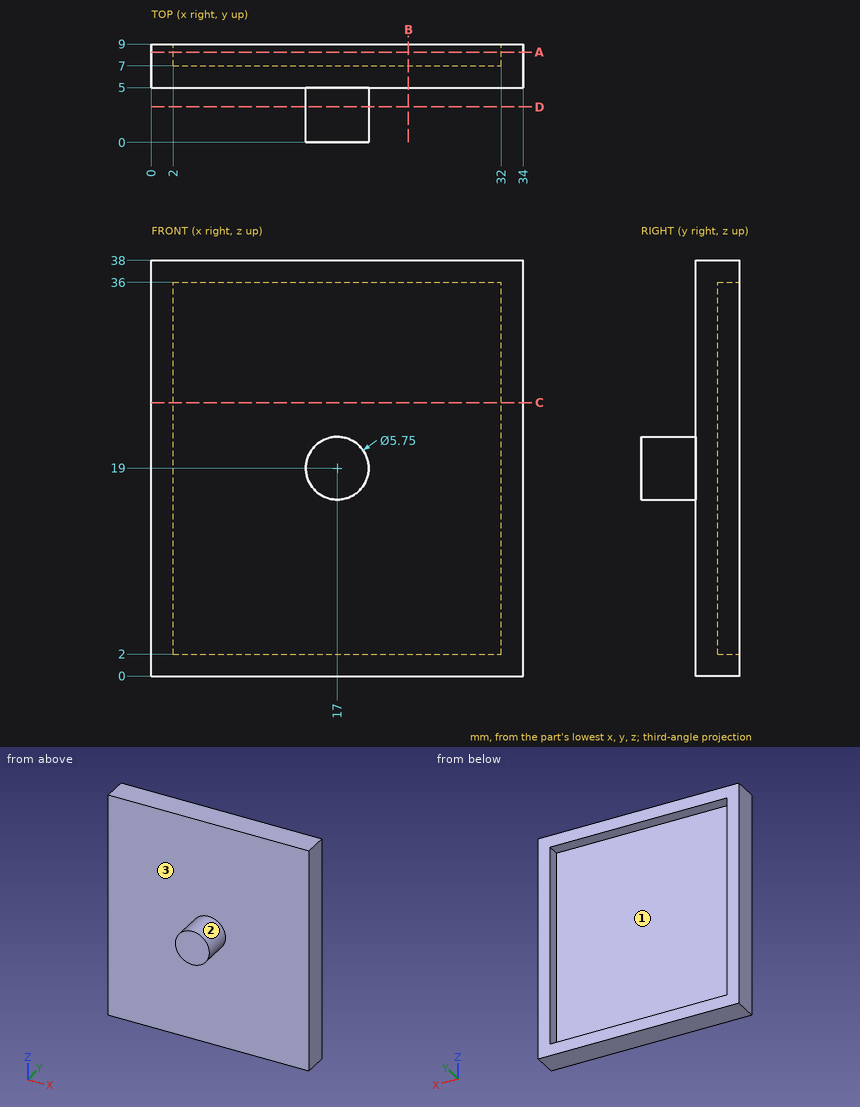
Geometry: see drawing. Coordinates: mm, zero at the bounding-box minimum. Give positions to 0.01 mm unless a question says otherwise; leave off trailing zeros. Loops run counter-clockwise (first coordinate to the right, second up) from the corner with the lowest first, then second, coordinate; pieces in that order, holes last. Notation, with made-up numbers: (-5, 24.25) - (46, 24.25) arc R28 cw to (46, 63.25) - close; hole circle Ø6 at (81, 29). An arc over 180 degrees is marked (long way). Use CSV: the item, a comma, the result in double quotes. Start each with the question number.
Item 1: Section C-C on z = 25. Return loops of the section in (x, y), then the cut area to 3 significant figures.
Item 2: Line query: line 1 (Z direction, x = 24, y = 8); line 2 (X direction, y = 8, z = 2.5); line 3 (Y direction, x = 27, z = 26.5). Output: solid intervals per line, ascending.
Item 3: Section D-D on y = 3.25. Return loops of the section in (x, z) (3 decimals).
Item 4: Section A-A on y = 8.25. Return loops of the section in (x, z), then the cut area to 3 significant figures.
Item 5: Contact query for flat-ended pins moving along their axis: P1, Ø3, axis at y = 2.5, z = 7, coming from the +X side; P2, Ø3, axis at x = 22, z = 11, coming from the -Y side. Output: stop coordinate, or through.
Item 6: Section B-B on x = 23.5. Return loops of the section in (y, z).
Item 7: Mould query, pull axis Z, two halves, no side actions, for the marked faces 1, 2 and 3. Classes: pulls with the +Z half, pulls with the -Z half, needs draft (parallel to the pull), parting line crosses it, or undercut.
Ans:
1,outline,"(0, 5) - (34, 5) - (34, 9) - (32, 9) - (32, 7) - (2, 7) - (2, 9) - (0, 9) - close"
1,area,"76.0 mm2"
2,line 1,"z = 0 to 2, 36 to 38"
2,line 2,"x = 0 to 2, 32 to 34"
2,line 3,"y = 5 to 7"
3,outline,"circle Ø5.75 at (17, 19)"
4,outline,"(0, 0) - (34, 0) - (34, 38) - (0, 38) - close; hole (2, 2) - (32, 2) - (32, 36) - (2, 36) - close"
4,area,"272 mm2"
5,P1,"passes through"
5,P2,"stops at y = 5"
6,outline,"(5, 0) - (9, 0) - (9, 2) - (7, 2) - (7, 36) - (9, 36) - (9, 38) - (5, 38) - close"
7,face 1,"undercut"
7,face 2,"parting line crosses it"
7,face 3,"needs draft"
